Geometry: final body of the model. Coordinates: model frame, mm. Give positions to 0.01 mm unless a question says otherwise; leave off trailing zeros. Order: outer loops, then holes, each group sorted by start corner. A loop starts at its lowest first (then second) coordinate and runs counter-clockwise, first axis right, second up. Notation, with made-up numbers: (23, -33) - (32, -33) arc R28 cw to (32, 1) - close; hole circle Ø1 at (19, 17). An arc over 180 degrees is marked (long way). One line per item, written item: value.
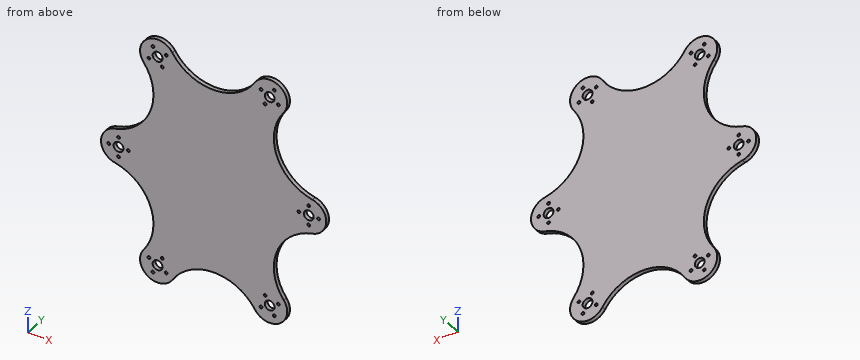
```python
from build123d import *

# Parameters (mm, degrees)
SKETCH2_R           = 3.5
SKETCH2_R_2         = 1
BOSS_EXTRUDE1_DEPTH = 3


with BuildPart() as part:
    # Sketch2 → Boss-Extrude1 (new body)
    with BuildSketch(Plane(origin=(0, 0, 0), x_dir=(1, 0, 0), z_dir=(0, 1, 0))):
        with BuildLine():
            ThreePointArc((-29.473684211, 81.741414978), (-47.137131817, 85.262131817), (-49.983079412, 67.477492077))
            ThreePointArc((-49.983079412, 67.477492077), (-45.123201765, 34.234985347), (-70.495895485, 12.214334182))
            ThreePointArc((-70.495895485, 12.214334182), (-80.338821814, 0), (-70.495895485, -12.214334182))
            ThreePointArc((-70.495895485, -12.214334182), (-45.123201765, -34.234985347), (-49.983079412, -67.477492077))
            ThreePointArc((-49.983079412, -67.477492077), (-47.137131817, -85.262131817), (-29.473684211, -81.741414978))
            ThreePointArc((-29.473684211, -81.741414978), (0, -65.617376915), (29.473684211, -81.741414978))
            ThreePointArc((29.473684211, -81.741414978), (47.137131817, -85.262131817), (49.983079412, -67.477492077))
            ThreePointArc((49.983079412, -67.477492077), (45.123201765, -34.234985347), (70.495895485, -12.214334182))
            ThreePointArc((70.495895485, -12.214334182), (80.338821814, 0), (70.495895485, 12.214334182))
            ThreePointArc((70.495895485, 12.214334182), (45.123201765, 34.234985347), (49.983079412, 67.477492077))
            ThreePointArc((49.983079412, 67.477492077), (47.137131817, 85.262131817), (29.473684211, 81.741414978))
            ThreePointArc((29.473684211, 81.741414978), (0, 65.617376915), (-29.473684211, 81.741414978))
        make_face()
        with Locations((-40, 75)):
            Circle(SKETCH2_R, mode=Mode.SUBTRACT)
        with Locations((-67.838821814, 0)):
            Circle(SKETCH2_R, mode=Mode.SUBTRACT)
        with Locations((-40, -75)):
            Circle(SKETCH2_R, mode=Mode.SUBTRACT)
        with Locations((40, -75)):
            Circle(SKETCH2_R, mode=Mode.SUBTRACT)
        with Locations((67.838821814, 0)):
            Circle(SKETCH2_R, mode=Mode.SUBTRACT)
        with Locations((40, 75)):
            Circle(SKETCH2_R, mode=Mode.SUBTRACT)
        with Locations((-36.705882353, 68.823529412)):
            Circle(SKETCH2_R_2, mode=Mode.SUBTRACT)
        with Locations((-33.823529412, 78.294117647)):
            Circle(SKETCH2_R_2, mode=Mode.SUBTRACT)
        with Locations((-43.294117647, 81.176470588)):
            Circle(SKETCH2_R_2, mode=Mode.SUBTRACT)
        with Locations((-46.176470588, 71.705882353)):
            Circle(SKETCH2_R_2, mode=Mode.SUBTRACT)
        with Locations((-36.705882353, -68.823529412)):
            Circle(SKETCH2_R_2, mode=Mode.SUBTRACT)
        with Locations((-33.823529412, -78.294117647)):
            Circle(SKETCH2_R_2, mode=Mode.SUBTRACT)
        with Locations((-43.294117647, -81.176470588)):
            Circle(SKETCH2_R_2, mode=Mode.SUBTRACT)
        with Locations((-46.176470588, -71.705882353)):
            Circle(SKETCH2_R_2, mode=Mode.SUBTRACT)
        with Locations((-60.838821814, 0)):
            Circle(SKETCH2_R_2, mode=Mode.SUBTRACT)
        with Locations((-67.838821814, 7)):
            Circle(SKETCH2_R_2, mode=Mode.SUBTRACT)
        with Locations((-67.838821814, -7)):
            Circle(SKETCH2_R_2, mode=Mode.SUBTRACT)
        with Locations((-74.838821814, 0)):
            Circle(SKETCH2_R_2, mode=Mode.SUBTRACT)
        with Locations((43.294117647, -81.176470588)):
            Circle(SKETCH2_R_2, mode=Mode.SUBTRACT)
        with Locations((33.823529412, -78.294117647)):
            Circle(SKETCH2_R_2, mode=Mode.SUBTRACT)
        with Locations((46.176470588, -71.705882353)):
            Circle(SKETCH2_R_2, mode=Mode.SUBTRACT)
        with Locations((36.705882353, -68.823529412)):
            Circle(SKETCH2_R_2, mode=Mode.SUBTRACT)
        with Locations((67.838821814, -7)):
            Circle(SKETCH2_R_2, mode=Mode.SUBTRACT)
        with Locations((60.838821814, 0)):
            Circle(SKETCH2_R_2, mode=Mode.SUBTRACT)
        with Locations((74.838821814, 0)):
            Circle(SKETCH2_R_2, mode=Mode.SUBTRACT)
        with Locations((67.838821814, 7)):
            Circle(SKETCH2_R_2, mode=Mode.SUBTRACT)
        with Locations((36.705882353, 68.823529412)):
            Circle(SKETCH2_R_2, mode=Mode.SUBTRACT)
        with Locations((46.176470588, 71.705882353)):
            Circle(SKETCH2_R_2, mode=Mode.SUBTRACT)
        with Locations((33.823529412, 78.294117647)):
            Circle(SKETCH2_R_2, mode=Mode.SUBTRACT)
        with Locations((43.294117647, 81.176470588)):
            Circle(SKETCH2_R_2, mode=Mode.SUBTRACT)
    extrude(amount=BOSS_EXTRUDE1_DEPTH)


solid = part.part
```
1) Section B-B, the plane z = -75. Return loops of the section in (x, y), then the cut area to 3 significant figures.
Answers below:
outline: (-52.5, 0) - (-43.5, 0) - (-43.5, 3) - (-52.5, 3) - close; (-36.5, 0) - (-23.85, 0) - (-23.85, 3) - (-36.5, 3) - close; (23.85, 0) - (36.5, 0) - (36.5, 3) - (23.85, 3) - close; (43.5, 0) - (52.5, 0) - (52.5, 3) - (43.5, 3) - close
area: 130 mm^2
2) Section C-C, the plane y = 1.4. Count the separate pieces of the cut face and the enclosed holes in it, then the cut area to 3 significant figures.
Answers below:
separate pieces: 1
enclosed holes: 30
area: 16,100 mm^2
3) Section A-A, the plane x = 40. Return loops of the section in (y, z), then the cut area to 3 significant figures.
Answers below:
outline: (0, -87.5) - (3, -87.5) - (3, -78.5) - (0, -78.5) - close; (0, -71.5) - (3, -71.5) - (3, 71.5) - (0, 71.5) - close; (0, 78.5) - (3, 78.5) - (3, 87.5) - (0, 87.5) - close
area: 483 mm^2
4) First-contact query: pin 1 (3 mm diameter, centred on x = 33.82, z = -78.29, fed in from +Y); pin 2 (1 mm diameter, centred on y = 1, z = 39, fed in from +X); pin 3 (1.8 mm diameter, centred on x = -33.82, z = 78.29, fed in from +Y). Flat tips, straight axial feed; report the tip coordinate or a pass-through.
Answers below:
pin 1: y = 3
pin 2: x = 43.84
pin 3: through
5) Section D-D, the plane x = -3. Return loops of the section in (y, z), then the cut area to 3 significant figures.
Answers below:
outline: (0, -65.75) - (3, -65.75) - (3, 65.75) - (0, 65.75) - close
area: 394 mm^2
6) Material intervals for line 1 along Z through (x, y) = (40, 2.05); line 2 along X through (y, z) = (1.5, 7); line 3 along Z through (x, y) = (42, 2.1), sorted ascending.
Answers below:
line 1: -87.5 to -78.5, -71.5 to 71.5, 78.5 to 87.5
line 2: -78.19 to -68.84, -66.84 to 66.84, 68.84 to 78.19
line 3: -87.34 to -77.87, -72.13 to 72.13, 77.87 to 87.34
